Autodesk Inventor part; units mm, degrees
ref_plane "YZ Plane" through (0, 0, 0) normal (1, 0, 0) x (0, 1, 0)
ref_plane "XZ Plane" through (0, 0, 0) normal (0, 1, 0) x (-1, 0, 0)
ref_plane "XY Plane" through (0, 0, 0) normal (0, 0, 1) x (1, 0, 0)
sketch "Sketch4" plane through (0, 0, 0) normal (0, 0, 1) x (1, 0, 0)
  line L0 (0, 0) -> (2.286, 0)
  line L1 (2.286, 0) -> (2.286, -25.4)
  line L2 (2.286, -25.4) -> (0, -25.4)
  line L3 (0, -25.4) -> (0, 0)
  line L4 (2.286, 0) -> (27.686, 0) construction
  line L5 (0.0779, 0.5917) -> (2.286, 0)
  arc A0 (0.0779, 0.5917) -> (0, 0) centre (2.286, 0) ccw
  line L6 (2.286, 0) -> (8.86, 24.5345)
  line L7 (2.286, 0) -> (27.686, 0) construction
  line L8 (8.86, 24.5345) -> (6.6519, 25.1262)
  line L9 (6.6519, 25.1262) -> (0.0779, 0.5917)
  dimension "d14" = 2.286
  dimension "d15" = 25.4
  dimension "d20" = 25.4
  dimension "d21" = 75
  dimension "d22" = 2.286
  dimension "d23" = 90
extrude "Extrusion2" add sketch "Sketch4" against normal blind 25.4
sketch "Sketch5" plane through (6.6519, 25.1262, -25.4) normal (-0.9659258, 0.258819, 0) x (0, 0, 1)
  line L0 (25.4, 0) -> (0, 0)
  line L1 (25.4, -25.4) -> (0, -25.4)
  point P0 (25.4, -25.9917)
  point P1 (12.7, -12.7)
  point P2 (12.7, 0)
  dimension "d26" = 12.7
sketch "Sketch6" plane through (0, -25.4, 0) normal (-1, 0, 0) x (0, 0, 1)
  line L0 (0, 0) -> (-25.4, 0)
  line L1 (0, 25.4) -> (-25.4, 25.4)
  point P0 (-12.7, 12.7)
  point P1 (-12.7, 0)
  dimension "d27" = 12.7
hole "Hole2" at (3.3649, 12.8589, -12.7) direction (0.9659258, -0.258819, 0) diameter 3.2512 end through all
hole "Hole3" at (0, -12.7, -12.7) direction (1, 0, 0) diameter 3.2512 end through all
fillet "Fillet2" radius 1.524 4 edges at (7.756, 24.8303, 0) (7.756, 24.8303, -25.4) (1.143, -25.4, -25.4) (1.143, -25.4, 0)
properties part number "am-2847" material "Steel"
Read the model definition and answer for the solid it produces. Units are mm, in the model's axes. A direction names the side the tool comes from. Round coordinates to 2 decimals unless told otherwise and drop trailing zeros. Write each loop counter-clockwise with the first axis right and the second up, starting at its lowest first coordinate (ties: lowest second). Pieces come first, ordered by that corner, then holes. Notation, with made-up numbers: (48, -25) - (84, -25) arc R16 cw to (84, 1) - close; hole circle Ø5 at (-15.75, 8). An arc over 180 degrees is marked (long way). Use a Markdown table: item, result.
(1) The part is cut by section C-C (z = -7). Write down the section's boundary in (x, y).
Reported:
| item | result |
|---|---|
| outline | (0, -25.4) - (2.29, -25.4) - (2.29, 0) - (8.86, 24.53) - (6.65, 25.13) - (0.08, 0.59) arc R2.29 ccw to (0, 0) - close |
(2) The part is cut by section B-B (z = -12.7). Write down the section's boundary in (x, y), then the cut area to 3 significant figures.
Reported:
| item | result |
|---|---|
| outline | (0, -25.4) - (2.29, -25.4) - (2.29, -14.33) - (0, -14.33) - close; (0, -11.07) - (2.29, -11.07) - (2.29, 0) - (5.15, 10.7) - (2.94, 11.29) - (0.08, 0.59) arc R2.29 ccw to (0, 0) - close; (3.79, 14.43) - (5.99, 13.84) - (8.86, 24.53) - (6.65, 25.13) - close |
| area | 102 mm2 |
(3) Straight lines are drawn through the part: line 1 along Z through (x, y) = (1.45, -12.7); line 2 along X through (y, z) = (-23, -12.5); line 3 along X through (y, z) = (2, -15.5). For each, find the intervals that lie inside material, in ascending order. Write a range as [from, to].
Reported:
| item | result |
|---|---|
| line 1 | [-25.4, -14.33], [-11.07, 0] |
| line 2 | [0, 2.29] |
| line 3 | [0.46, 2.82] |
(4) The mould has two halves that part along Y. Classify faces 3 (the cylindrical face through (4.36, 12.09, -11.15)), 4 (the cylindrical face through (7.628, 24.415, -24.942)), 5 (the flat face through (2, 0, -25.4)), 6 (the cylindrical face through (1.159, -12.077, -11.198)): released by +Y, released by -Y, zero draft, split by the parting line, or undercut.
Reported:
| item | result |
|---|---|
| face 3 | undercut |
| face 4 | released by +Y |
| face 5 | zero draft |
| face 6 | undercut |
(5) Which of the six approach directions +Z, -Z, +X, -X, +Y, -Y give full straight-line access (tool end or side, diameter ignored) to faces 1 (the flat face through (4.141, 15.757, -12.522)), 2 (the flat face through (2.286, -15, -13))?
Reported:
| item | result |
|---|---|
| face 1 | +Z, -Z, -X, +Y |
| face 2 | +Z, -Z, +X, -Y |
(6) Each of these flat-tipped pins is pushed along its axis until it touches: pin 1 Ø7.5 at (y, z) = (-11, -16) entering from +X; pin 2 Ø2 at (y, z) = (-12.7, -12.7) entering from -X; pin 3 Ø1 at (x, z) = (2.5, -4.5) entering from -Y. Where does it stop, or does it pass through?
Reported:
| item | result |
|---|---|
| pin 1 | x = 2.29 |
| pin 2 | through |
| pin 3 | y = -25.4 |
(7) The part is cut by section D-D (x = 1.25). Write down the section's boundary in (y, z).
Reported:
| item | result |
|---|---|
| outline | (-25.4, -23.88) arc R1.52 ccw to (-23.88, -25.4) - (4.97, -25.4) - (4.97, 0) - (-23.88, 0) arc R1.52 ccw to (-25.4, -1.52) - close; hole circle Ø3.25 at (-12.7, -12.7) |
(8) The part is cut by section A-A (y = -12.7). Write down the section's boundary in (x, z), then the cut area to 3 significant figures.
Reported:
| item | result |
|---|---|
| outline | (0, -25.4) - (2.29, -25.4) - (2.29, -14.33) - (0, -14.33) - close; (0, -11.07) - (2.29, -11.07) - (2.29, 0) - (0, 0) - close |
| area | 50.6 mm2 |
